CAD build for the part. Positions are in the model's coordinates, mm. Face numbers are marked on the shaded views. A direction names the side the tool comes from. Give positions to 0.01 mm unless a question says otherwise; leave off trailing zeros. Write each loop counter-clockwise with the first axis right and the second up, starting at its lowest first coordinate (ties: lowest second). Pieces come first, ordered by that corner, then holes. Notation, with made-up numbers: (-32, 53) -> (3, 53) arc R4 ccw to (3, 57) -> close; hole circle Ø1 at (77, -12). An arc over 180 degrees is marked (long way). Answer as a JSON object with one key per item and string values.
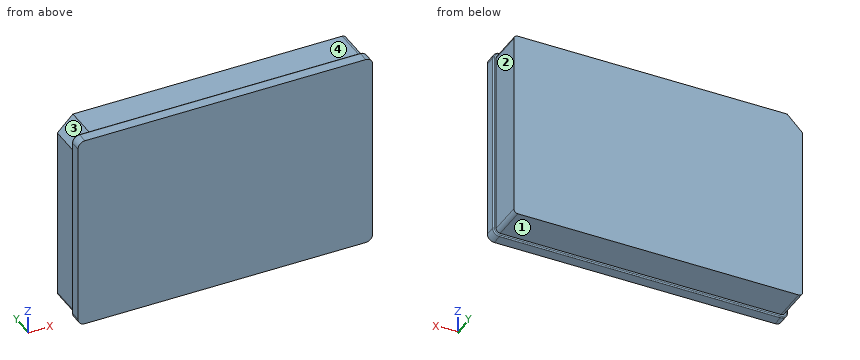
```python
from build123d import *

# Parameters (mm, degrees)
SKETCH1_W           = 127.75
SKETCH1_H           = 85.6
BOSS_EXTRUDE1_DEPTH = 20
FILLET1_R           = 3
CUT_EXTRUDE2_DEPTH  = 15
FILLET5_R           = 0.5


with BuildPart() as part:
    # Sketch1 → Boss-Extrude1 (new body)
    with BuildSketch(Plane(origin=(0, 0, 0), x_dir=(1, 0, 0), z_dir=(0, 1, 0))):
        Rectangle(SKETCH1_W, SKETCH1_H)
    extrude(amount=BOSS_EXTRUDE1_DEPTH)

    # Fillet1
    fillet1_edges = [part.edges().sort_by_distance(p)[0] for p in [
        (-63.875, 10, -42.8),
        (63.875, 10, -42.8),
        (63.875, 10, 42.8),
        (-63.875, 10, 42.8),
    ]]
    fillet(fillet1_edges, radius=FILLET1_R)

    # Sketch3 → Cut-Extrude2 (cut)
    with BuildSketch(Plane(origin=(0, 20, 0), x_dir=(1, 0, 0), z_dir=(0, 1, 0))):
        with BuildLine():
            Line((-63.875, 39.8), (-63.875, -39.8))
            ThreePointArc((-63.875, -39.8), (-62.996320344, -41.921320344), (-60.875, -42.8))
            Line((-60.875, -42.8), (60.875, -42.8))
            ThreePointArc((60.875, -42.8), (62.996320344, -41.921320344), (63.875, -39.8))
            Line((63.875, -39.8), (63.875, 39.8))
            ThreePointArc((63.875, 39.8), (62.996320344, 41.921320344), (60.875, 42.8))
            Line((60.875, 42.8), (-60.875, 42.8))
            ThreePointArc((-60.875, 42.8), (-62.996320344, 41.921320344), (-63.875, 39.8))
        make_face()
        with BuildLine():
            Line((-62.625, 39.8), (-62.625, -34.8))
            Line((-62.625, -34.8), (-55.875, -41.55))
            Line((-55.875, -41.55), (60.875, -41.55))
            ThreePointArc((60.875, -41.55), (62.112436867, -41.037436867), (62.625, -39.8))
            Line((62.625, -39.8), (62.625, 39.8))
            ThreePointArc((62.625, 39.8), (62.112436867, 41.037436867), (60.875, 41.55))
            Line((60.875, 41.55), (-60.875, 41.55))
            ThreePointArc((-60.875, 41.55), (-62.112436867, 41.037436867), (-62.625, 39.8))
        make_face(mode=Mode.SUBTRACT)
    extrude(amount=-CUT_EXTRUDE2_DEPTH, mode=Mode.SUBTRACT)

    # Fillet5
    fillet5_edges = [part.edges().sort_by_distance(p)[0] for p in [
        (-62.996320344, 5, -41.921320344),
        (0, 5, -42.8),
        (62.996320344, 5, -41.921320344),
        (63.875, 5, 0),
        (62.996320344, 5, 41.921320344),
        (0, 5, 42.8),
        (-62.996320344, 5, 41.921320344),
        (-63.875, 5, 0),
    ]]
    fillet(fillet5_edges, radius=FILLET5_R)


solid = part.part
```
1) Pin check, flat tips, straight feed: pin 1 (12 mm diameter, centred on y = 15.5, z = -7, fed in from +X) (3 decimals); pin 2 (10 mm diameter, centred on x = 8, y = 11, fed in from -Z); pin 3 (4.5 mm diameter, centred on x = -10, y = 13.5, fed in from +Z). Stop position of each tip, or through.
Model answer:
{"pin 1": "stops at x = 62.625", "pin 2": "stops at z = -41.55", "pin 3": "stops at z = 41.55"}
2) Wall check: probe 1 along X at (y, z) = (12.5, 31) (3 decimals); probe 2 along Z at (x, y) = (38.5, 9); probe 3 along X at (y, z) = (11, 37) (3 decimals). Give the ranges that are in metal, low to high.
Model answer:
{"probe 1": "x = -62.625 to 62.625", "probe 2": "z = -41.55 to 41.55", "probe 3": "x = -60.425 to 62.625"}
3) Slice it at A-A (x = 53). List the corners of the cut face in (y, z), then the cut area to 3 significant figures.
Model answer:
{"outline": "(0, -42.8) -> (4.5, -42.8) arc R0.5 ccw to (5, -42.3) -> (5, -41.55) -> (20, -41.55) -> (20, 41.55) -> (5, 41.55) -> (5, 42.3) arc R0.5 ccw to (4.5, 42.8) -> (0, 42.8) -> close", "area": "1,670 mm2"}
4) Slice it at B-B (y = 12). List the corners of the cut face in (x, z) (3 decimals), then the cut area to 3 significant figures.
Model answer:
{"outline": "(-62.625, -39.8) arc R1.75 ccw to (-60.875, -41.55) -> (60.875, -41.55) arc R1.75 ccw to (62.625, -39.8) -> (62.625, 39.8) arc R1.75 ccw to (60.875, 41.55) -> (-55.875, 41.55) -> (-62.625, 34.8) -> close", "area": "10,400 mm2"}
5) 3-axis set-ups, long thin cutter, end or side, ignore diameter. For the marked faces 1, 2, 3 and 4: which of +Z, -Z, +X, -X, +Y, -Y reach the whole face in a straight line?
Model answer:
{"face 1": "-Z, +X, -X, +Y", "face 2": "+Z, -Z, +X, +Y", "face 3": "+Z, -X, +Y", "face 4": "+Z, +X, -X, +Y"}
